Here's how the part is built. I have some questions about the finished solid (model axes, mm). Face numbers are marked on the shaded views. A direction names the side the tool comes from. Coordinates: 2 decimals unless noted, no trailing zeros. Write each loop counter-clockwise with the first axis right and the second up, starting at its lowest first coordinate (ties: lowest second). Pieces come first, ordered by that corner, then holes.
Item 1: For the marked faces 1, 2 and 3, which set-ups out of +Z, -Z, +X, -X, +Y, -Y let a thin tool reach every point of the face, with its end or its side?
Item 2: I'm going to push flat-ended pins straight in: P1, Ø1.9, axis at x = 27.5, z = 2, coming from the -Y side; P2, Ø10, axis at x = 55, z = 29.5, coming from the +Y side; P3, Ø2.5, axis at x = 73, z = 37.5, coming from the +Y side. Where does each tip first touch, or does it pass through?
Item 3: I want a section at C-C (y = 11.5). Please give me the cut outline in (x, z) (3 decimals).
Item 4: I want a section at B-B (x = 40). Please give me the cut outline in (y, z) (3 decimals), and give its area (3 significant figures).
Item 5: I want a section at A-A (y = -26). Please give me the cut outline in (x, z) (3 decimals), and give its area (3 significant figures).
Item 6: I want a section at D-D (z = 28). Please give me the cut outline in (x, y), and give its area (3 significant figures).
Item 7: Please list where these lines run through material, in increasing order: line 1 (Z direction, x = 63.5, y = 20.5) (3 decimals); line 2 (Z direction, x = 27.5, y = -20) (3 decimals); line 3 (Y direction, x = 56, z = 30).
from build123d import *

# Parameters (mm, degrees)
PAD_DEPTH = 100


with BuildPart() as part:
    # Sketch → Pad (new body)
    with BuildSketch(Plane.YZ):
        Polygon((-30.04999, 0), (29.988436, 0), (29.988436, 6.484765), (4.088979, 6.484765), (4.088979, 35.272057), (29.985703, 35.272057), (29.985703, 39.984997), (-30.064808, 39.984997), (-30.064808, 35.199318), (-4.016708, 35.199318), (-4.016708, 6.430613), (-30.04999, 6.430613), align=None)
    extrude(amount=PAD_DEPTH)


solid = part.part
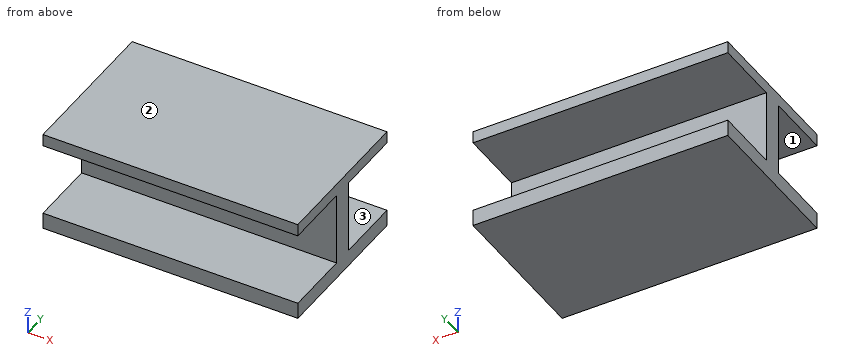
Answer:
1. face 1: +X, -X, -Y
1. face 2: +Z, +X, -X, +Y, -Y
1. face 3: +X, -X, +Y
2. P1: stops at y = -30.05
2. P2: stops at y = 4.09
2. P3: stops at y = 29.99
3. outline: (0, 0) - (100, 0) - (100, 6.485) - (0, 6.485) - close; (0, 35.272) - (100, 35.272) - (100, 39.985) - (0, 39.985) - close
4. outline: (-30.065, 35.199) - (-4.017, 35.199) - (-4.017, 6.431) - (-30.05, 6.431) - (-30.05, 0) - (29.988, 0) - (29.988, 6.485) - (4.089, 6.485) - (4.089, 35.272) - (29.986, 35.272) - (29.986, 39.985) - (-30.065, 39.985) - close
4. area: 906 mm2
5. outline: (0, 0) - (100, 0) - (100, 6.431) - (0, 6.431) - close; (0, 35.199) - (100, 35.199) - (100, 39.985) - (0, 39.985) - close
5. area: 1,120 mm2
6. outline: (0, -4.02) - (100, -4.02) - (100, 4.09) - (0, 4.09) - close
6. area: 811 mm2
7. line 1: z = 0 to 6.485, 35.272 to 39.985
7. line 2: z = 0 to 6.431, 35.199 to 39.985
7. line 3: y = -4.02 to 4.09
